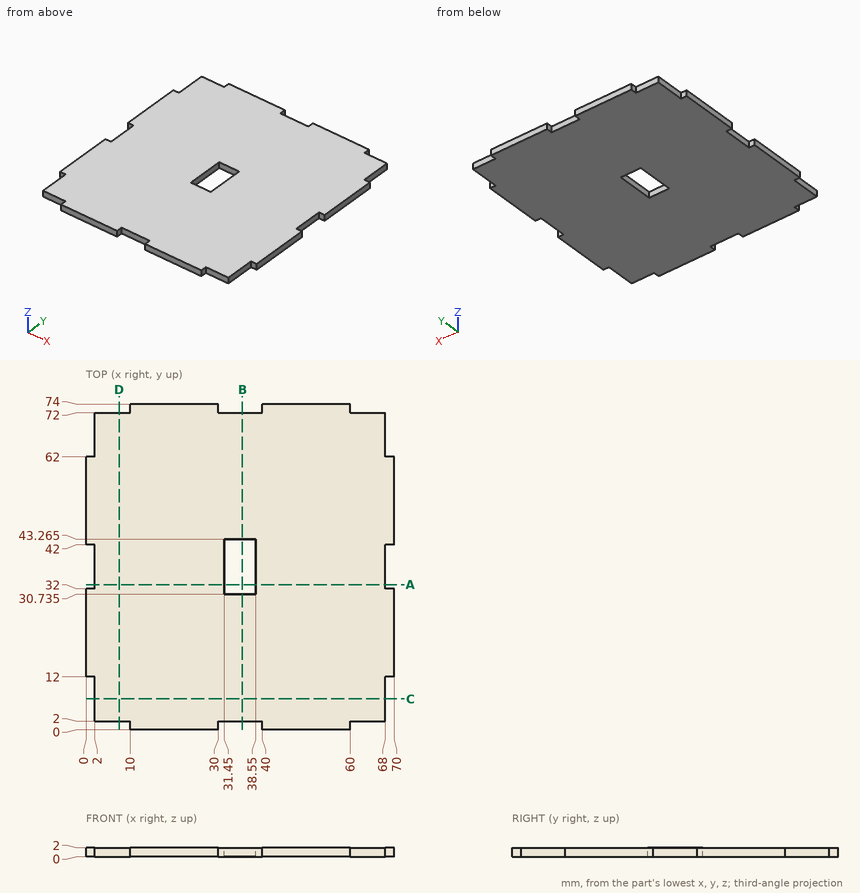
The drawing under review shows one solid part. Ordinate dimensions are in mm from its lowest x, y, z. Coordinates: 2 decimals unless noted, no trailing zeros. Order: outer loops, then holes, each group sorted by start corner. A loop starts at its lowest first (then second) coordinate and runs counter-clockwise, first axis right, second up. Notation, with made-up numbers: (-19.75, -10.5) -> (5.25, -10.5) arc R22 ccw to (5.25, 0.5) -> close; hole circle Ø8 at (9.25, -26). An arc over 180 degrees is marked (long way). Answer in a Markdown table with one row per item. Add a question column.
Item 1: We need section B-B on x = 35.5. Write out the cut boundary in (y, z) (3 decimals).
Item 2: Clearance check with flat-ended pins moving along their axes: pin 1 (1 mm diameter, centred on y = 39, z = 0.5, fed in from +X); pin 2 (0.6 mm diameter, centred on x = 1, z = 1, fed in from -Y); pin 3 (0.6 mm diameter, centred on y = 0.5, z = 1.5, fed in from +X). State where each tip first meets the part, or that it passes through.
Item 3: We need section C-C on y = 7. Write out the cut boundary in (x, z), plus the area to 3 significant figures.
Item 4: We need section D-D on x = 7.5. Write out the cut boundary in (y, z), plus the area to 3 significant figures.
Item 5: We need section A-A on y = 33. Write out the cut boundary in (x, z).
Item 6: To check wall thickness, follow probe 1 along Y at (x, z) = (34, 0.85) (3 decimals); probe 2 along X at (y, z) = (63, 1.7); probe 3 along Y at (x, z) = (5.5, 0.35). State the ranges of each line that lie inside material, in increasing order.
Final values:
| question | item | result |
|---|---|---|
| 1 | outline | (2, 0) -> (30.735, 0) -> (30.735, 2) -> (2, 2) -> close; (43.265, 0) -> (72, 0) -> (72, 2) -> (43.265, 2) -> close |
| 2 | pin 1 | stops at x = 68 |
| 2 | pin 2 | stops at y = 12 |
| 2 | pin 3 | stops at x = 60 |
| 3 | outline | (2, 0) -> (68, 0) -> (68, 2) -> (2, 2) -> close |
| 3 | area | 132 mm2 |
| 4 | outline | (2, 0) -> (72, 0) -> (72, 2) -> (2, 2) -> close |
| 4 | area | 140 mm2 |
| 5 | outline | (2, 0) -> (31.45, 0) -> (31.45, 2) -> (2, 2) -> close; (38.55, 0) -> (68, 0) -> (68, 2) -> (38.55, 2) -> close |
| 6 | probe 1 | y = 2 to 30.735, 43.265 to 72 |
| 6 | probe 2 | x = 2 to 68 |
| 6 | probe 3 | y = 2 to 72 |
